```python
from build123d import *

# Parameters (mm, degrees)
MAIN_SPAR_DEPTH                                = 3
T_TABS_TOP_PLATE_DEPTH                         = 3
LONG_TAB_DEPTH                                 = 3
SKETCH2_W                                      = 3.2
SKETCH2_H                                      = 31
TAB_SLOTS_DEPTH                                = 182.612802412
TAB_SLOT_EXTRA_RELIEF_AND_CABLE_CLEARANC_REACH = 183.613
SKETCH9_W                                      = 13.1
SKETCH9_H                                      = 15.75
SIDE_PLATE_SLOT_DEPTH                          = 182.612802412
ELASTIC_ANCHORS_REACH                          = 183.613


with BuildPart() as part:
    # Sketch1 → main spar (new body)
    with BuildSketch(Plane.XY):
        with BuildLine():
            Line((-29.5, 171), (29.5, 171))
            Line((29.5, 171), (29.5, 108))
            ThreePointArc((29.5, 108), (30.112758667, 104.92938679), (31.857166371, 102.329159794))
            Line((31.857166371, 102.329159794), (57.642833629, 76.670840206))
            ThreePointArc((57.642833629, 76.670840206), (59.387241333, 74.07061321), (60, 71))
            Line((60, 71), (60, 63))
            Line((60, 63), (0, 63))
            Line((0, 63), (-60, 63))
            Line((-60, 63), (-60, 71))
            ThreePointArc((-60, 71), (-59.387241333, 74.07061321), (-57.642833629, 76.670840206))
            Line((-57.642833629, 76.670840206), (-31.857166371, 102.329159794))
            ThreePointArc((-31.857166371, 102.329159794), (-30.112758667, 104.92938679), (-29.5, 108))
            Line((-29.5, 108), (-29.5, 171))
        make_face()
    extrude(amount=MAIN_SPAR_DEPTH)

    # Sketch10 → T tabs top plate (add)
    with BuildSketch(Plane(origin=(0, 0, 0), x_dir=(-1, 0, 0), z_dir=(0, 0, -1))):
        with BuildLine():
            Line((53.5, 63), (53.5, 55.616234023))
            ThreePointArc((53.5, 55.616234023), (57.740053742, 53.859946258), (55.983765977, 58.1))
            Line((55.983765977, 58.1), (55, 58.1))
            Line((55, 58.1), (55, 60.1))
            Line((55, 60.1), (58, 60.1))
            ThreePointArc((58, 60.1), (60.621768891, 53.985808943), (54.750795687, 50.857122632))
            ThreePointArc((54.750795687, 50.857122632), (53.887952488, 50.679903583), (53.5, 49.88908259))
            Line((53.5, 49.88908259), (53.5, 47.88908259))
            Line((53.5, 47.88908259), (38.5, 47.88908259))
            Line((38.5, 47.88908259), (38.5, 49.88908259))
            ThreePointArc((38.5, 49.88908259), (38.112047512, 50.679903583), (37.249204313, 50.857122632))
            ThreePointArc((37.249204313, 50.857122632), (31.378231109, 53.985808943), (34, 60.1))
            Line((34, 60.1), (37, 60.1))
            Line((37, 60.1), (37, 58.1))
            Line((37, 58.1), (36.016234023, 58.1))
            ThreePointArc((36.016234023, 58.1), (34.259946258, 53.859946258), (38.5, 55.616234023))
            Line((38.5, 55.616234023), (38.5, 63))
            Line((38.5, 63), (30.9, 63))
            Line((30.9, 63), (30.9, 65))
            Line((30.9, 65), (61.1, 65))
            Line((61.1, 65), (61.1, 63))
            Line((61.1, 63), (53.5, 63))
        make_face()
        with BuildLine():
            Line((-38.5, 63), (-38.5, 55.616234023))
            ThreePointArc((-38.5, 55.616234023), (-34.259946258, 53.859946258), (-36.016234023, 58.1))
            Line((-36.016234023, 58.1), (-37, 58.1))
            Line((-37, 58.1), (-37, 60.1))
            Line((-37, 60.1), (-34, 60.1))
            ThreePointArc((-34, 60.1), (-31.378231109, 53.985808943), (-37.249204313, 50.857122632))
            ThreePointArc((-37.249204313, 50.857122632), (-38.112047512, 50.679903583), (-38.5, 49.88908259))
            Line((-38.5, 49.88908259), (-38.5, 47.88908259))
            Line((-38.5, 47.88908259), (-53.5, 47.88908259))
            Line((-53.5, 47.88908259), (-53.5, 49.88908259))
            ThreePointArc((-53.5, 49.88908259), (-53.887952488, 50.679903583), (-54.750795687, 50.857122632))
            ThreePointArc((-54.750795687, 50.857122632), (-60.621768891, 53.985808943), (-58, 60.1))
            Line((-58, 60.1), (-55, 60.1))
            Line((-55, 60.1), (-55, 58.1))
            Line((-55, 58.1), (-55.983765977, 58.1))
            ThreePointArc((-55.983765977, 58.1), (-57.740053742, 53.859946258), (-53.5, 55.616234023))
            Line((-53.5, 55.616234023), (-53.5, 63))
            Line((-53.5, 63), (-61.1, 63))
            Line((-61.1, 63), (-61.1, 65))
            Line((-61.1, 65), (-30.9, 65))
            Line((-30.9, 65), (-30.9, 63))
            Line((-30.9, 63), (-38.5, 63))
        make_face()
    extrude(amount=-T_TABS_TOP_PLATE_DEPTH)

    # Sketch11 → long tab (add)
    with BuildSketch(Plane(origin=(0, 0, 0), x_dir=(-1, 0, 0), z_dir=(0, 0, -1))):
        Polygon((32, 47.88908259), (60, 47.88908259), (60, 3), (53.5, 3), (53.5, -0.3), (56.5, -0.3), (56.5, -3.3), (35.5, -3.3), (35.5, -0.3), (38.5, -0.3), (38.5, 3), (32, 3), align=None)
        Polygon((-60, 47.88908259), (-32, 47.88908259), (-32, 3), (-38.5, 3), (-38.5, -0.3), (-35.5, -0.3), (-35.5, -3.3), (-56.5, -3.3), (-56.5, -0.3), (-53.5, -0.3), (-53.5, 3), (-60, 3), align=None)
    extrude(amount=-LONG_TAB_DEPTH)

    # Sketch2 → tab slots (cut, through all)
    with BuildSketch(Plane.XY.offset(3)):
        with Locations((12, 140.5)):
            Rectangle(SKETCH2_W, SKETCH2_H)
        with Locations((-12, 140.5)):
            Rectangle(SKETCH2_W, SKETCH2_H)
        with BuildLine():
            Line((10.3, 72), (7.3, 72))
            Line((7.3, 72), (7.3, 78))
            ThreePointArc((7.3, 78), (6.55, 78.75), (5.8, 78))
            Line((5.8, 78), (5.8, 57))
            Line((5.8, 57), (13.5, 57))
            Line((13.5, 57), (13.5, 72))
            Line((13.5, 72), (13.5, 85.108254278))
            ThreePointArc((13.5, 85.108254278), (14.330080695, 86.38576104), (12.935889894, 87))
            Line((12.935889894, 87), (10.935889894, 87))
            ThreePointArc((10.935889894, 87), (9.55273068, 86.420438505), (10.3, 85.120204103))
            Line((10.3, 85.120204103), (10.3, 74))
            ThreePointArc((10.3, 74), (10.9, 73), (10.3, 72))
        make_face()
        with BuildLine():
            Line((-10.3, 72), (-7.3, 72))
            Line((-7.3, 72), (-7.3, 78))
            ThreePointArc((-7.3, 78), (-6.55, 78.75), (-5.8, 78))
            Line((-5.8, 78), (-5.8, 57))
            Line((-5.8, 57), (-13.5, 57))
            Line((-13.5, 57), (-13.5, 72))
            Line((-13.5, 72), (-13.5, 85.108254278))
            ThreePointArc((-13.5, 85.108254278), (-14.330080695, 86.38576104), (-12.935889894, 87))
            Line((-12.935889894, 87), (-10.935889894, 87))
            ThreePointArc((-10.935889894, 87), (-9.55273068, 86.420438505), (-10.3, 85.120204103))
            Line((-10.3, 85.120204103), (-10.3, 74))
            ThreePointArc((-10.3, 74), (-10.9, 73), (-10.3, 72))
        make_face()
    extrude(amount=-TAB_SLOTS_DEPTH, mode=Mode.SUBTRACT)

    # Sketch9 → tab slot extra relief and cable clearanc (cut, up to next)
    with BuildSketch(Plane.XY.offset(3), mode=Mode.PRIVATE) as tab_slot_extra_relief_and_cable_clearanc_sk1:
        with Locations((0, 70.875)):
            Rectangle(SKETCH9_W, SKETCH9_H)
    tab_slot_extra_relief_and_cable_clearanc_tool1 = extrude(tab_slot_extra_relief_and_cable_clearanc_sk1.sketch, amount=-TAB_SLOT_EXTRA_RELIEF_AND_CABLE_CLEARANC_REACH, mode=Mode.PRIVATE) & part.part
    add(tab_slot_extra_relief_and_cable_clearanc_tool1.solids().sort_by_distance((0, 70.875, 3))[0], mode=Mode.SUBTRACT)

    # Sketch4 → side plate slot (cut, through all)
    with BuildSketch(Plane.XY.offset(3)):
        Polygon((-60, 35), (-54.39, 35), (-54.39, 41), (-51.19, 41), (-51.19, 10), (-60, 10), align=None)
    side_plate_slot = extrude(amount=-SIDE_PLATE_SLOT_DEPTH, mode=Mode.SUBTRACT)

    # side plate slot mirror: side plate slot across plane
    add(side_plate_slot.mirror(Plane(origin=(0, 0, 0), x_dir=(0, 0, 1), z_dir=(1, 0, 0))), mode=Mode.SUBTRACT)

    # Sketch8 → elastic anchors (cut, up to next)
    with BuildSketch(Plane.XY.offset(3), mode=Mode.PRIVATE) as elastic_anchors_sk1:
        with BuildLine():
            ThreePointArc((22.96414143, 158.500428674), (24.060660172, 161.060660172), (21.500428674, 159.96414143))
            ThreePointArc((21.500428674, 159.96414143), (18.304532331, 162.662597854), (21.178026712, 165.702079807))
            ThreePointArc((21.178026712, 165.702079807), (24.986612172, 165.166705802), (28.5, 163.602079807))
            ThreePointArc((28.5, 163.602079807), (32.25852471, 160.13767164), (34.5, 155.543716867))
            Line((34.5, 155.543716867), (34.5, 177.660442747))
            ThreePointArc((34.5, 177.660442747), (32.25852471, 173.066487973), (28.5, 169.602079807))
            ThreePointArc((28.5, 169.602079807), (24.986612172, 168.037453812), (21.178026712, 167.502079807))
            ThreePointArc((21.178026712, 167.502079807), (16.589455886, 161.913585252), (22.96414143, 158.500428674))
        make_face()
    elastic_anchors_tool1 = extrude(elastic_anchors_sk1.sketch, amount=-ELASTIC_ANCHORS_REACH, mode=Mode.PRIVATE) & part.part
    # Sketch8 → elastic anchors (cut, up to next)
    with BuildSketch(Plane.XY.offset(3), mode=Mode.PRIVATE) as elastic_anchors_sk2:
        with BuildLine():
            ThreePointArc((22.96414143, 128.500428674), (24.060660172, 131.060660172), (21.500428674, 129.96414143))
            ThreePointArc((21.500428674, 129.96414143), (18.304532331, 132.662597854), (21.178026712, 135.702079807))
            ThreePointArc((21.178026712, 135.702079807), (24.986612172, 135.166705802), (28.5, 133.602079807))
            ThreePointArc((28.5, 133.602079807), (32.25852471, 130.13767164), (34.5, 125.543716867))
            Line((34.5, 125.543716867), (34.5, 147.660442747))
            ThreePointArc((34.5, 147.660442747), (32.25852471, 143.066487973), (28.5, 139.602079807))
            ThreePointArc((28.5, 139.602079807), (24.986612172, 138.037453812), (21.178026712, 137.502079807))
            ThreePointArc((21.178026712, 137.502079807), (16.589455886, 131.913585252), (22.96414143, 128.500428674))
        make_face()
    elastic_anchors_tool2 = extrude(elastic_anchors_sk2.sketch, amount=-ELASTIC_ANCHORS_REACH, mode=Mode.PRIVATE) & part.part
    # Sketch8 → elastic anchors (cut, up to next)
    with BuildSketch(Plane.XY.offset(3), mode=Mode.PRIVATE) as elastic_anchors_sk3:
        with BuildLine():
            ThreePointArc((-22.96414143, 128.500428674), (-24.060660172, 131.060660172), (-21.500428674, 129.96414143))
            ThreePointArc((-21.500428674, 129.96414143), (-18.304532331, 132.662597854), (-21.178026712, 135.702079807))
            ThreePointArc((-21.178026712, 135.702079807), (-24.986612172, 135.166705802), (-28.5, 133.602079807))
            ThreePointArc((-28.5, 133.602079807), (-32.25852471, 130.13767164), (-34.5, 125.543716867))
            Line((-34.5, 125.543716867), (-34.5, 147.660442747))
            ThreePointArc((-34.5, 147.660442747), (-32.25852471, 143.066487973), (-28.5, 139.602079807))
            ThreePointArc((-28.5, 139.602079807), (-24.986612172, 138.037453812), (-21.178026712, 137.502079807))
            ThreePointArc((-21.178026712, 137.502079807), (-16.589455886, 131.913585252), (-22.96414143, 128.500428674))
        make_face()
    elastic_anchors_tool3 = extrude(elastic_anchors_sk3.sketch, amount=-ELASTIC_ANCHORS_REACH, mode=Mode.PRIVATE) & part.part
    # Sketch8 → elastic anchors (cut, up to next)
    with BuildSketch(Plane.XY.offset(3), mode=Mode.PRIVATE) as elastic_anchors_sk4:
        with BuildLine():
            ThreePointArc((-22.96414143, 158.500428674), (-24.060660172, 161.060660172), (-21.500428674, 159.96414143))
            ThreePointArc((-21.500428674, 159.96414143), (-18.304532331, 162.662597854), (-21.178026712, 165.702079807))
            ThreePointArc((-21.178026712, 165.702079807), (-24.986612172, 165.166705802), (-28.5, 163.602079807))
            ThreePointArc((-28.5, 163.602079807), (-32.25852471, 160.13767164), (-34.5, 155.543716867))
            Line((-34.5, 155.543716867), (-34.5, 177.660442747))
            ThreePointArc((-34.5, 177.660442747), (-32.25852471, 173.066487973), (-28.5, 169.602079807))
            ThreePointArc((-28.5, 169.602079807), (-24.986612172, 168.037453812), (-21.178026712, 167.502079807))
            ThreePointArc((-21.178026712, 167.502079807), (-16.589455886, 161.913585252), (-22.96414143, 158.500428674))
        make_face()
    elastic_anchors_tool4 = extrude(elastic_anchors_sk4.sketch, amount=-ELASTIC_ANCHORS_REACH, mode=Mode.PRIVATE) & part.part
    add(elastic_anchors_tool1.solids().sort_by_distance((27.986566, 165.492974, 3))[0], mode=Mode.SUBTRACT)
    add(elastic_anchors_tool2.solids().sort_by_distance((27.986566, 135.492974, 3))[0], mode=Mode.SUBTRACT)
    add(elastic_anchors_tool3.solids().sort_by_distance((-27.986566, 135.492974, 3))[0], mode=Mode.SUBTRACT)
    add(elastic_anchors_tool4.solids().sort_by_distance((-27.986566, 165.492974, 3))[0], mode=Mode.SUBTRACT)


solid = part.part
```
For this review, take the finished solid that the model builds, in its own axes (mm). A direction names the side the tool comes from. Give positions to 0.01 mm unless a question says otherwise; leave off trailing zeros. Loops run counter-clockwise (first coordinate to the right, second up) from the corner with the lowest first, then second, coordinate; pieces in that order, holes last. Notation, with made-up numbers: M 23,-30 L 58,-30 A22 cw 58,-1 Z; hole C -26,60 d7. An arc over 180 degrees is marked long. One line per item, written item: value. Start each with the question number.
Q1. Machinability: for faces 1 (the face through (-18.31, 162.6, 1.52)), 2 (the face through (-1, 85, 0)), which of the approach directions +Z, -Z, +X, -X, +Y, -Y give a long, thin tool a straight path to every point of the face, cutting with its end or side? Answer none if there is none.
Q2. Draft analysis for pull direction Y (two halves, no side actions). For faces 3 (the face through (44.57, 89.68, 1.48)), 4 (the face through (18.31, 162.6, 1.52)), 5 (the face through (-1, 85, 3)), state which applies: released by +Y, released by -Y, zero draft, split by the parting line, or undercut.
Q3. For L1, parallel to X at y = 86.1, z = 0.75; L2, parallel to X at y = 8, z = 2.6; L3, parallel to Y at x = 20, z = 1.15, list the stretches that pass through material, from the lowest coordinate up.
Q4. Add section A-A (y = 27.5). Give the boundary of the cut face in (x, z), and give its area (3 significant figures).
Q5. Add section B-B (x = -47.5). Give the boundary of the cut face in (y, z), and give its area (3 significant figures).
Q6. Clearance check with flat-ended pins moving along their axes: pin 1 Ø0.9 at (y, z) = (35, 2) entering from +X; pin 2 Ø1.5 at (y, z) = (130, 2) entering from -X; pin 3 Ø0.9 at (x, z) = (55, 1.5) entering from +Y. State where each tip first meets the part, or that it passes through.
Q7. Add section C-C (z = 0.6). Count the separate pieces of the cut face and the enclosed holes in it, and give its area (3 significant figures).
Q8. Add section D-D (x = 42). Give the boundary of the cut face in (y, z), and give its area (3 significant figures).
Reply:
1. face 1: +Z, -Z
1. face 2: -Z, +X, -X, +Y, -Y
2. face 3: released by +Y
2. face 4: undercut
2. face 5: zero draft
3. L1: -48.17 to -14.37, -9.5 to 9.5, 14.37 to 48.17
3. L2: -60 to -32, 32 to 60
3. L3: 63 to 128.3, 130.2 to 135.45, 137.35 to 158.3, 160.2 to 165.45, 167.35 to 171
4. outline: M -51.19,0 L -32,0 L -32,3 L -51.19,3 Z; M 32,0 L 51.19,0 L 51.19,3 L 32,3 Z
4. area: 115 mm²
5. outline: M -3.3,0 L 86.76,0 L 86.76,3 L -3.3,3 Z
5. area: 270 mm²
6. pin 1: x = 60
6. pin 2: x = -29.5
6. pin 3: y = 79.75
7. separate pieces: 1
7. enclosed holes: 2
7. area: 9,980 mm²
8. outline: M -3.3,0 L 92.24,0 L 92.24,3 L -3.3,3 Z
8. area: 287 mm²
